Autodesk Inventor part; units mm, degrees
ref_plane "YZ Plane" through (0, 0, 0) normal (1, 0, 0) x (0, 1, 0)
ref_plane "XZ Plane" through (0, 0, 0) normal (0, 1, 0) x (-1, 0, 0)
ref_plane "XY Plane" through (0, 0, 0) normal (0, 0, 1) x (1, 0, 0)
sketch "Sketch1" plane through (0, 0, 0) normal (0, 0, 1) x (1, 0, 0)
  line L0 (6.6074, 9.0814) -> (61.6074, 9.0814)
  line L1 (61.6074, 9.0814) -> (61.6074, 16.0814)
  line L2 (52.6074, 19.0814) -> (6.6074, 19.0814)
  line L3 (6.6074, 19.0814) -> (6.6074, 9.0814)
  line L4 (52.6074, 16.0814) -> (52.6074, 19.0814)
  line L5 (52.6074, 16.0814) -> (61.6074, 16.0814)
  point P0 (0, 0)
  dimension "d0" = 55
  dimension "d1" = 7
  dimension "d6" = 9
  dimension "d7" = 3
extrude "Extrusion1" add sketch "Sketch1" along normal blind 70
sketch "Sketch2" plane through (6.6074, 19.0814, 0) normal (0, 1, 0) x (1, 0, 0)
  circle A0 centre (23, -10) radius 4
  circle A1 centre (23, -60) radius 4
  line L0 (46, -70) -> (0, -70)
  line L1 (55, 0) -> (55, -70)
  line L2 (46, 0) -> (0, 0)
  circle A2 centre (30, -35) radius 8
  line L3 (55, 0) -> (55, -70)
  circle A3 centre (50.5, -60) radius 3
  line L4 (46, 0) -> (46, -70)
  line L5 (55, -70) -> (46, -70)
  circle A4 centre (50.5, -41.5) radius 3
  circle A5 centre (50.5, -10) radius 3
  circle A6 centre (50.5, -28.5) radius 3
  line L6 (55, 0) -> (46, 0)
  line L7 (30, -43) -> (12.7252, -43)
  line L8 (23, -56) -> (14.0477, -56)
  line L9 (9, -14) -> (9, -56)
  line L10 (9, -56) -> (51, -56)
  line L11 (51, -56) -> (51, -14)
  line L12 (51, -14) -> (9, -14)
  circle A7 centre (14.5, -19.5) radius 2
  circle A8 centre (45.5, -19.5) radius 2
  circle A9 centre (45.5, -50.5) radius 2
  circle A10 centre (14.5, -51.5) radius 2
  line L13 (1, -101.1728) -> (51, -101.1728)
  circle A11 centre (39, -60) radius 2
  circle A12 centre (7, -60) radius 2
  circle A13 centre (30, -35) radius 12.5
  circle A14 centre (7, -60) radius 4
  circle A15 centre (39, -60) radius 4
  line L14 (0, 0) -> (0, -70)
  line L15 (0, -35) -> (-6.6074, -35)
  circle A16 centre (39, -10) radius 2
  circle A17 centre (7, -10) radius 2
  circle A18 centre (7, -10) radius 4
  circle A19 centre (39, -10) radius 4
  line L16 (37, -60) -> (37, -51.6268)
  line L17 (35, -60) -> (35, -52.1291)
  circle A20 centre (23, -60) radius 9
  line L18 (11, -60) -> (11, -66.8543)
  line L19 (14, -60) -> (14, -67.7509)
  line L20 (32, -60) -> (32, -67.7509)
  circle A21 centre (23, -60) radius 10
  line L21 (13, -60) -> (13, -90.2082)
  circle A22 centre (7, -97.0024) radius 2
  line L22 (13, -90.2082) -> (13, -105.086)
  circle A23 centre (39, -97.0024) radius 2
  line L23 (51, -101.1728) -> (51, -88.3214)
  line L24 (33, -60) -> (33, -163.1603)
  line L25 (1, -101.1728) -> (1, -81.8849)
  circle A24 centre (50.5, -105.086) radius 6.5
  line L26 (43, -90.2082) -> (43, -98.586)
  point P0 (-6.6074, 0)
  dimension "d11" = 8
  dimension "d17" = 16
  dimension "d55" = 4
  dimension "d64" = 8
  dimension "d65" = 8
  dimension "d10" = 8
  dimension "d12" = 10
  dimension "d15" = 10
  dimension "d18" = 35
  dimension "d22" = 6
  dimension "d23" = 4.5
  dimension "d24" = 10
  dimension "d30" = 10
  dimension "d33" = 32
  dimension "d34" = 32
  dimension "d35" = 25
  dimension "d36" = 4.5
  dimension "d37" = 4.5
  dimension "d40" = 42
  dimension "d41" = 42
  dimension "d42" = 42
  dimension "d43" = 4
  dimension "d44" = 4
  dimension "d45" = 4
  dimension "d46" = 4
  dimension "d47" = 31
  dimension "d48" = 31
  dimension "d50" = 32
  dimension "d51" = 5.5
  dimension "d52" = 5.5
  dimension "d53" = 5.5
  dimension "d54" = 50
  dimension "d56" = 4
  dimension "d59" = 60
  dimension "d60" = 60
  dimension "d61" = 21
  dimension "d62" = 5.5
  dimension "d63" = 25
  dimension "d69" = 7
  dimension "d71" = 18
  dimension "d72" = 14
  dimension "d73" = 14
  dimension "d74" = 20
  dimension "d75" = 4
  dimension "d76" = 4
  dimension "d79" = 6
  dimension "d80" = 6
  dimension "d83" = 12
  dimension "d84" = 13
  dimension "d86" = 8
  dimension "d129" = 28.5
  dimension "d130" = 28.5
extrude "Extrusion2" cut sketch "Sketch2" against normal blind 30 contours A0 | L11 A6 | A6 L11 | A1 | L11 A4 | A4 L11 | A2 | A3 | A5
sketch "Sketch4" plane through (6.6074, 9.0814, 0) normal (0, -1, 0) x (1, 0, 0)
  circle A0 centre (7, 60) radius 2
  circle A1 centre (39, 60) radius 2
  circle A2 centre (7, 10) radius 2
  circle A3 centre (39, 10) radius 2
  dimension "d97" = 4
  dimension "d98" = 4
  dimension "d99" = 4
extrude "Extrusion4" cut sketch "Sketch4" against normal blind 70
sketch "Boceto5" plane through (6.6074, 9.0814, 0) normal (-1, 0, 0) x (0, 0, 1)
  circle A0 centre (38.25, 7) radius 1
  circle A1 centre (31.75, 7) radius 1
  line L0 (70, 10) -> (70, 0)
  line L1 (0, 10) -> (70, 10)
  line L2 (35, 6.1177) -> (35, -0.846)
  point P0 (0, -9.0814)
  dimension "d106" = 2
  dimension "d139" = 3
  dimension "d140" = 2
  dimension "d141" = 3
  dimension "d142" = 6.5
  dimension "d143" = 3.25
  dimension "d144" = 35
hole "Agujero1" at (6.6074, 16.0814, 38.25) at (6.6074, 16.0814, 31.75) direction (1, 0, 0) diameter 2 depth 15 tip angle 120
thread "Thread3"
thread "Thread4"
thread "Thread5"
thread "Thread6"
thread "Thread7"
thread "Thread8"
chamfer "Chaflán1" distance 1 angle 45 1 edges at (52.6074, 19.0814, 35)
properties part number "Techo, Vínculo Cabezal" material "Aluminum 6061"
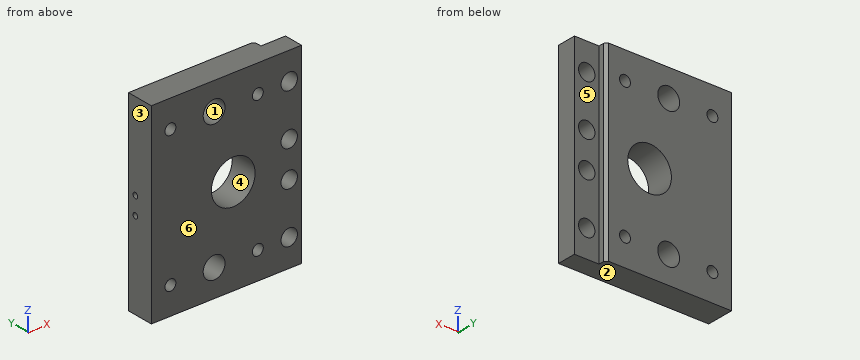
Design review of the part built by this model. Coordinates are the model's own, in mm. Face numbers are marked on the shaded views. A direction names the side the tool comes from. Coordinates: 2 decimals unless noted, no trailing zeros. Order: outer loops, then holes, each group sorted by start corner. A loop starts at its lowest first (then second) coordinate and runs counter-clockwise, first axis right, second up. Notation, with made-up numbers: (-6, 12) -> (53, 12) arc R21 ccw to (53, 40) -> close; hole circle Ø11 at (26.5, 89). An arc over 180 degrees is marked (long way). Use one line per item in the form item = value. Start each with the question number.
(1) For probe 1 along Z at (x, y) = (59, 15.25); probe 2 along Z at (x, y) = (28.5, 12); probe 3 along Z at (x, y) = (26.5, 11), list the stretches that pass through material, from the lowest coordinate up.
(2) Add section D-D on z = 28.5. State the section outline as (x, y) points.
(3) Add section B-B on z = 60. State the section outline as (x, y) points, plus the area to 4 significant figures.
(4) For the marked faces 5 and 6, list the 3-axis set-ups (+Z, -Z, +X, -X, +Y, -Y) from which the entire face can be reached by the end or side of a thin tool; tool diameter is ignored.
(5) Add section C-C on x = 39.5. State the section outline as (y, z) points, plus the area to 3 significant figures.
(6) Insertion check: pin 1 (3.5 mm diameter, centred on x = 57.11, z = 28.5, fed in from +Y); pin 2 (4.5 mm diameter, centred on x = 56, z = 48, fed in from +Y). Each pin has a flat end and moves straight along its axis. Give the tip position at first contact, or say it passes through.
(7) Add section A-A on y = 13.75. Give the number of separate pieces and of enclosed holes in the cut face, plus the area to 3 significant figures.
(8) The part is to be moulded in two halves that separate along Z. For the marked faces 1, 2, 3 and 4, say which applies: +Z half, -Z half, draft (parallel to the pull), parting line (faces both ways), or undercut.
Answer block:
q1.probe_1 = 0 to 7.67, 12.33 to 26.17, 30.83 to 39.17, 43.83 to 57.67, 62.33 to 70
q1.probe_2 = 0 to 6.16, 13.84 to 56.16, 63.84 to 70
q1.probe_3 = 0 to 7.48, 12.52 to 57.48, 62.52 to 70
q2.outline = (6.61, 9.08) -> (31.94, 9.08) -> (31.94, 19.08) -> (6.61, 19.08) -> close; (41.27, 9.08) -> (54.11, 9.08) -> (54.11, 16.08) -> (52.61, 16.08) -> (52.61, 18.08) -> (51.61, 19.08) -> (41.27, 19.08) -> close; (60.11, 9.08) -> (61.61, 9.08) -> (61.61, 16.08) -> (60.11, 16.08) -> close
q3.outline = (6.61, 9.08) -> (11.61, 9.08) -> (11.61, 19.08) -> (6.61, 19.08) -> close; (15.61, 9.08) -> (25.61, 9.08) -> (25.61, 19.08) -> (15.61, 19.08) -> close; (33.61, 9.08) -> (43.61, 9.08) -> (43.61, 19.08) -> (33.61, 19.08) -> close; (47.61, 9.08) -> (54.11, 9.08) -> (54.11, 16.08) -> (52.61, 16.08) -> (52.61, 18.08) -> (51.61, 19.08) -> (47.61, 19.08) -> close; (60.11, 9.08) -> (61.61, 9.08) -> (61.61, 16.08) -> (60.11, 16.08) -> close
q3.area = 320.5 mm²
q4.face_5 = +Z, -Z, +X, +Y
q4.face_6 = +Z, -Z, +X, -X, -Y
q5.outline = (9.08, 0) -> (19.08, 0) -> (19.08, 27.54) -> (9.08, 27.54) -> close; (9.08, 42.46) -> (19.08, 42.46) -> (19.08, 70) -> (9.08, 70) -> close
q5.area = 551 mm²
q6.pin_1 = through
q6.pin_2 = 16.08
q7.separate_pieces = 1
q7.enclosed_holes = 11
q7.area = 3,390 mm²
q8.face_1 = undercut
q8.face_2 = -Z half
q8.face_3 = draft
q8.face_4 = undercut
